Geometry check sheet. Reference: the model listing, model coordinates, mm. A direction names the side the tool comes from. Give positions to 0.01 mm unless a question says otherwise; leave off trailing zeros. Loops run counter-clockwise (first coordinate to the right, second up) from the corner with the lowest first, then second, coordinate; pieces in that order, holes last. Notation, with made-up numbers: (-25, -28) -> (-5, -28) arc R18 ccw to (-5, -11) -> close; hole circle Ø8 at (43.25, -25). An arc over 180 degrees is marked (long way). One line per item, written item: value. Start each with the question number.
(1) Draft check along X on faces 3 (the face through (779.55, -2114.61, 4.93)), 4 (the face through (823.95, -2081.71, 4.93)), 5 (the face through (890.418, -2223.625, 4.93)), 6 (the face through (987, -2034, 0)). Enter one of: pulls with the +X half, pulls with the -X half, needs draft (parallel to the pull), parting line crosses it, or undercut.
(2) Gauge pin test, flat ends, axial feed: pin 1 Ø3 at (y, z) = (-2252.5, 8.5) entering from +X; pin 2 Ø5 at (x, z) = (945, 2.5) entering from +Y; pin 3 Ø6 at (y, z) = (-2027, 6.5) entering from +X; pin 4 Ø5 at (x, y) = (1257, -1986.5) entering from -Z. Record the tip position at first contact, or that the pin passes through.
(3) Tool access check on faces 1 (the face through (671.838, -1807.906, 4.93)), 2 (the face through (1137.188, -1790.985, 4.93)). Record the directions out of +Z, -Z, +X, -X, +Y, -Y that give a thin tool (end or side, any length) a straight path to the whole face; none if there is none.
(4) Scan lines: line 1 along X through (y, z) = (-1962, 3.5); line 2 along Y through (x, z) = (841.5, 3); line 3 along Y through (x, z) = (821, 1.75). Record each from-to range of solid material in increasing order. Write a range as from..to.
(5) Sectioned sample at B-B, the plane z = 2.5. State how many separate pieces and enclosed holes the cut face has, then the cut area to 3 significant figures.
(6) Sectioned sample at C-C, the plane x = 694. Record the cut outline in (y, z).
(7) Sectioned sample at A-A, the plane y = -2187.5. Record the cut outline in (x, z).
from build123d import *

# Parameters (mm, degrees)
MODEL_R            = 2
MODEL_W            = 19.645816046
MODEL_H            = 39.291293686
BOSS_EXTRU_1_DEPTH = 10


with BuildPart() as part:
    # Model → Boss.-Extru.1 (new body)
    with BuildSketch(Plane.XY):
        with BuildLine():
            Line((682.695045286, -1946.855082062), (879.151513744, -2287.127966132))
            add(Edge.make_bspline(
                [(879.151513744, -2287.127966132), (889.999791642, -2305.917615253), (883.561957827, -2329.943588049), (864.772308706, -2340.79203515)],
                knots=[1, 1, 1, 1, 2, 2, 2, 2], degree=3))
            Line((864.772308706, -2340.79203515), (879.080786919, -2365.574852737))
            Line((879.080786919, -2365.574852737), (909.407369941, -2365.574852737))
            Line((909.407369941, -2365.574852737), (1075.393432839, -2365.574852737))
            Line((1075.393432839, -2365.574852737), (1105.720015861, -2365.574852737))
            Line((1105.720015861, -2365.574852737), (1120.02849407, -2340.792035147))
            add(Edge.make_bspline(
                [(1120.02849407, -2340.792035147), (1101.238844947, -2329.94358805), (1094.801011127, -2305.917615255), (1105.649289021, -2287.127966132)],
                knots=[7, 7, 7, 7, 8, 8, 8, 8], degree=3))
            Line((1105.649289021, -2287.127966132), (1302.105757418, -1946.855082026))
            add(Edge.make_bspline(
                [(1302.105757418, -1946.855082026), (1312.954035312, -1928.065432904), (1336.980177311, -1921.627768287), (1355.769826434, -1932.475876978)],
                knots=[9, 9, 9, 9, 10, 10, 10, 10], degree=3))
            Line((1355.769826434, -1932.475876978), (1370.178134382, -1907.519964771))
            Line((1370.178134382, -1907.519964771), (1355.114672609, -1881.429377608))
            Line((1355.114672609, -1881.429377608), (1271.929088191, -1737.347990137))
            Line((1271.929088191, -1737.347990137), (1256.886607583, -1711.292935573))
            Line((1256.886607583, -1711.292935573), (1228.035135874, -1711.292935573))
            add(Edge.make_bspline(
                [(1228.035135874, -1711.292935573), (1228.035135876, -1732.992875424), (1210.443782043, -1750.58422926), (1188.743842192, -1750.584229262)],
                knots=[17, 17, 17, 17, 18, 18, 18, 18], degree=3))
            Line((1188.743842192, -1750.584229262), (795.830566931, -1750.584229262))
            add(Edge.make_bspline(
                [(795.830566931, -1750.584229262), (774.13062708, -1750.584229264), (756.539273244, -1732.992875431), (756.539273242, -1711.29293558)],
                knots=[19, 19, 19, 19, 20, 20, 20, 20], degree=3))
            Line((756.539273242, -1711.29293558), (727.617413106, -1711.29293558))
            Line((727.617413106, -1711.29293558), (614.474446531, -1907.262945538))
            Line((614.474446531, -1907.262945538), (629.030976268, -1932.475877023))
            add(Edge.make_bspline(
                [(629.030976268, -1932.475877023), (647.820625389, -1921.627599125), (671.846767389, -1928.065432941), (682.695045286, -1946.855082062)],
                knots=[23, 23, 23, 23, 24, 24, 24, 24], degree=3))
        make_face()
        with Locations((716.491657861, -1754.205060963)):
            Circle(MODEL_R, mode=Mode.SUBTRACT)
        with Locations((645.852191539, -1876.556374988)):
            Circle(MODEL_R, mode=Mode.SUBTRACT)
        with Locations((921.760877273, -2353.746974362)):
            Circle(MODEL_R, mode=Mode.SUBTRACT)
        with Locations((1063.039925504, -2353.746974349)):
            Circle(MODEL_R, mode=Mode.SUBTRACT)
        with Locations((1338.602199082, -1876.556405894)):
            Circle(MODEL_R, mode=Mode.SUBTRACT)
        with Locations((1267.962617169, -1754.205060913)):
            Circle(MODEL_R, mode=Mode.SUBTRACT)
        Polygon((1223.175627189, -1950.912568739), (1262.446954927, -1952.164332155), (1261.821242422, -1971.799996024), (1222.549576279, -1970.548232608), align=None, mode=Mode.SUBTRACT)
        Polygon((1168.677387646, -2107.576225944), (1134.756257166, -2087.748009122), (1144.67053478, -2070.787443882), (1178.59166526, -2090.615660704), align=None, mode=Mode.SUBTRACT)
        Polygon((1146.688110722, -1773.475865452), (1163.955948518, -1782.84480196), (1145.218413907, -1817.380308349), (1127.950576111, -1808.011541044), align=None, mode=Mode.SUBTRACT)
        Polygon((1085.080978488, -2205.721381517), (1105.440492577, -2239.326440884), (1088.637962894, -2249.506197929), (1068.278448805, -2215.901138562), align=None, mode=Mode.SUBTRACT)
        with Locations((992.287035365, -1805.015464432)):
            Rectangle(MODEL_W, MODEL_H, mode=Mode.SUBTRACT)
        Polygon((900.740118048, -2206.587700635), (917.542647733, -2216.767457676), (897.18313365, -2250.372517047), (880.380603964, -2240.192760005), align=None, mode=Mode.SUBTRACT)
        Polygon((836.808814024, -1773.475865479), (855.54634864, -1808.011541068), (838.278510846, -1817.380308376), (819.540976229, -1782.844801991), align=None, mode=Mode.SUBTRACT)
        Polygon((841.150900137, -2071.65376301), (851.065177754, -2088.614328248), (817.144047278, -2108.442545076), (807.229769661, -2091.481979838), align=None, mode=Mode.SUBTRACT)
        Polygon((762.645807706, -1951.778887881), (763.271520215, -1971.41455175), (724.000192478, -1972.666315173), (723.374479969, -1953.030651304), align=None, mode=Mode.SUBTRACT)
    extrude(amount=BOSS_EXTRU_1_DEPTH)


solid = part.part
Calculated:
1. face 3: pulls with the -X half
1. face 4: undercut
1. face 5: undercut
1. face 6: needs draft
2. pin 1: stops at x = 1126.51
2. pin 2: stops at y = -1750.58
2. pin 3: stops at x = 1257.57
2. pin 4: stops at z = 0
3. face 1: +Z, -Z, -X, +Y
3. face 2: +Z, -Z
4. line 1: x = 691.44..723.66, 762.97..1222.82, 1262.13..1293.36
4. line 2: y = -2221.91..-2094.21, -2072.25..-1815.63, -1782.12..-1750.58
4. line 3: y = -2186.41..-2106.19, -2083.43..-1785.53, -1782.05..-1750.58
5. separate pieces: 1
5. enclosed holes: 15
5. area: 290,000 mm2
6. outline: (-1966.44, 0) -> (-1769.52, 0) -> (-1769.52, 10) -> (-1966.44, 10) -> close
7. outline: (821.63, 0) -> (1163.17, 0) -> (1163.17, 10) -> (821.63, 10) -> close
